Source: CAD feature listing. Evaluate the final solid. Frame: model axes, mm. A direction names the side the tool comes from. Give positions to 0.01 mm unless a question says otherwise; leave off trailing zeros. Loops run counter-clockwise (first coordinate to the right, second up) from the corner with the lowest first, then second, coordinate; pieces in that order, holes last.
```python
from build123d import *

# Parameters (mm, degrees)
F0_R     = 2.5
F0_R_2   = 6
F1_DEPTH = 5
F2_W     = 2
F2_H     = 10
F3_DEPTH = 7.3521866209
F4_SIZE  = 1


with BuildPart() as f1:
    # F0 (on Top) → F1 (new body, symmetric)
    with BuildSketch(Plane.XY):
        with BuildLine():
            ThreePointArc((-16.05, 4.3757856437), (-19.5, 0), (-16.05, -4.3757856437))
            Line((-16.05, -4.3757856437), (-1.8666666667, -7.7791744778))
            ThreePointArc((-1.8666666667, -7.7791744778), (-0.9398415233, -7.9446018095), (0, -8))
            ThreePointArc((0, -8), (0.9398415233, -7.9446018095), (1.8666666667, -7.7791744778))
            Line((1.8666666667, -7.7791744778), (16.05, -4.3757856437))
            ThreePointArc((16.05, -4.3757856437), (19.5, 0), (16.05, 4.3757856437))
            Line((16.05, 4.3757856437), (4, 7.267266404))
            Line((4, 7.267266404), (4, 13.267266404))
            Line((4, 13.267266404), (0, 13.267266404))
            Line((0, 13.267266404), (-4, 13.267266404))
            Line((-4, 13.267266404), (-4, 7.267266404))
            Line((-4, 7.267266404), (-16.05, 4.3757856437))
        make_face()
        with Locations((-15, 0)):
            Circle(F0_R, mode=Mode.SUBTRACT)
        Circle(F0_R_2, mode=Mode.SUBTRACT)
        with Locations((15, 0)):
            Circle(F0_R, mode=Mode.SUBTRACT)
    extrude(amount=F1_DEPTH, both=True)

    # F2 (on face) → F3 (cut, through all)
    with BuildSketch(Plane(origin=(0, 13.267266404, 0), x_dir=(-1, 0, 0), z_dir=(0, 1, 0))):
        Rectangle(F2_W, F2_H)
    extrude(amount=-F3_DEPTH, mode=Mode.SUBTRACT)

    # F4
    f4_edges = [f1.edges().sort_by_distance(p)[0] for p in [
        (-4, 13.267266, 0),
        (4, 13.267266, 0),
    ]]
    chamfer(f4_edges, length=F4_SIZE)


solid = f1.part
```
(1) Mould query, pull axis Y, two halves, no side actions, for faces 5 (the cylindrical face through (19.5, -0.1, 0.1)), 6 (the flat face through (3, 6, 5)), 7 (the cylindrical face through (-17.5, 0.1, -0.1)), 8 (the cylindrical face through (0, -6, 0)). Classes: pulls with the +Y half, pulls with the -Y half, needs draft (parallel to the pull), parting line crosses it, or undercut.
A:
face 5: parting line crosses it
face 6: needs draft
face 7: undercut
face 8: undercut
(2) First-contact query: pin 1 (2 mm diameter, centred on y = 11, z = 1, fed in from -X); pin 2 (1 mm diameter, centred on y = -2.5, z = 0.5, fed in from -X); pin 3 (1.5 mm diameter, centred on y = 10.5, z = -2, fed in from +X). Flat tips, straight axial feed; report the tip coordinate or a pass-through.
A:
pin 1: stops at x = -4
pin 2: stops at x = -19.03
pin 3: stops at x = 4
(3) Section D-D, the plane x = 15. Return the cut outline in (y, z).
A:
outline: (-4.63, -5) - (-2.5, -5) - (-2.5, 5) - (-4.63, 5) - close; (2.5, -5) - (4.63, -5) - (4.63, 5) - (2.5, 5) - close
(4) Section A-A, the plane y = 10.25. Return the cut outline in (x, z).
A:
outline: (-4, -5) - (-1, -5) - (-1, 5) - (-4, 5) - close; (1, -5) - (4, -5) - (4, 5) - (1, 5) - close
(5) Ray query, line 1 along X through (y, z) = (8.75, -0.5); line 2 along X through (y, z) = (-1.75, -1); line 3 along X through (y, z) = (0.5, 3.5). Return the intervals inside material, ascending.
A:
line 1: x = -4 to -1, 1 to 4
line 2: x = -19.15 to -16.79, -13.21 to -5.74, 5.74 to 13.21, 16.79 to 19.15
line 3: x = -19.47 to -17.45, -12.55 to -5.98, 5.98 to 12.55, 17.45 to 19.47
(6) Reachability of faces 1 (the flat face through (-4, 10, 0)), 2 (the flat face through (1, 10, 0)), 3 (the flat face through (8.86, -6.1, 0.07)), 4 (the flat face through (4, 10, 0)) from +Z, -Z, +X, -X, +Y, -Y: full face, straight path, thin tool, end or side. Return the list, or none.
A:
face 1: +Z, -Z, -X, +Y
face 2: +Z, -Z, +Y
face 3: +Z, -Z, +X, -Y
face 4: +Z, -Z, +X, +Y
(7) Section C-C, the plane z = 0. Return the cut outline in (x, y), then the cut area to 3 significant figures.
A:
outline: (-16.05, -4.38) - (-1.87, -7.78) arc R8 ccw to (1.87, -7.78) - (16.05, -4.38) arc R4.5 ccw to (16.05, 4.38) - (4, 7.27) - (4, 12.27) - (3, 13.27) - (1, 13.27) - (1, 5.92) arc R6 cw (long way) to (-1, 5.92) - (-1, 13.27) - (-3, 13.27) - (-4, 12.27) - (-4, 7.27) - (-16.05, 4.38) arc R4.5 ccw to start; hole circle Ø5 at (-15, 0); hole circle Ø5 at (15, 0)
area: 325 mm2
(8) Section B-B, the plane y = 0. Return the cut outline in (x, z), then the cut area to 3 significant figures.
A:
outline: (-19.5, -5) - (-17.5, -5) - (-17.5, 5) - (-19.5, 5) - close; (-12.5, -5) - (-6, -5) - (-6, 5) - (-12.5, 5) - close; (6, -5) - (12.5, -5) - (12.5, 5) - (6, 5) - close; (17.5, -5) - (19.5, -5) - (19.5, 5) - (17.5, 5) - close
area: 170 mm2
